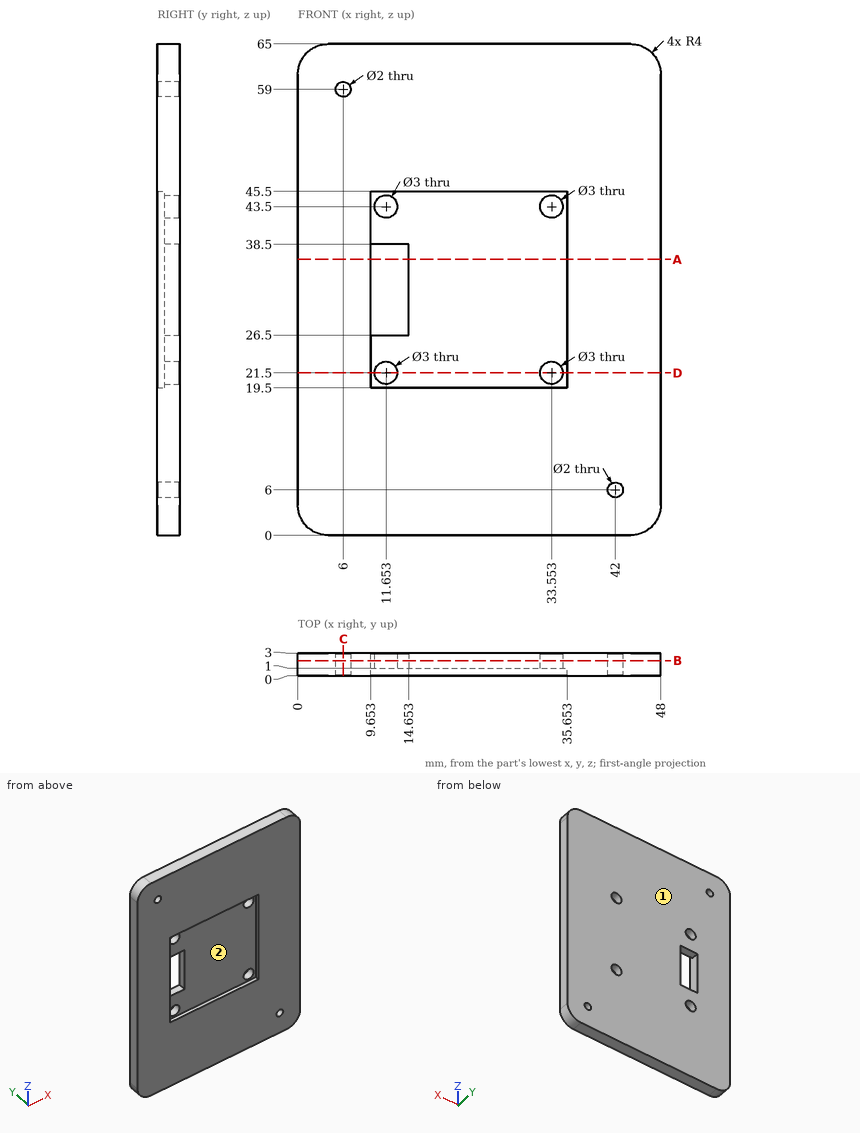
The figure shows three views and two pictorial views of one solid part (mm, origin at its lowest corner). Answer the questions. Give positions to 0.01 mm unless a question says otherwise; leave off trailing zeros. Loops run counter-clockwise (first coordinate to the right, second up) from the corner with the lowest first, then second, coordinate; pieces in that order, holes last. Notation, with made-up numbers: (71, 41) -> (81, 41) arc R23 ccw to (81, 50) -> close; hole circle Ø7 at (-15, 87). An arc over 180 degrees is marked (long way). Use a Markdown table: item, result. Add a question column.
1. Section C-C on x = 6 is taken. Determine the outline of the cut face in (y, z).
2. Section A-A on z = 36.5 is taken. Determine the outline of the cut face in (x, y).
3. Section B-B on y = 2.05 is taken. Determine the outline of the cut face in (x, z).
4. Section D-D on z = 21.5 is taken. Determine the outline of the cut face in (x, y).
5. Find the intervals of material crossed by probe 1 along X at (y, z) = (1.85, 43.5); probe 2 along Z at (x, y) = (42, 1.95); probe 3 along X at (y, z) = (0.95, 22.5), in increasing order.
6. Determine the mould class of the marked faces 1 and 2 for opening direction Z: released by +Z, released by -Z, zero draft, split by the parting line, or undercut.
Results below:
| question | item | result |
|---|---|---|
| 1 | outline | (0, 0) -> (3, 0) -> (3, 58) -> (0, 58) -> close; (0, 60) -> (3, 60) -> (3, 65) -> (0, 65) -> close |
| 2 | outline | (0, 0) -> (9.65, 0) -> (9.65, 3) -> (0, 3) -> close; (14.65, 1) -> (35.65, 1) -> (35.65, 0) -> (48, 0) -> (48, 3) -> (14.65, 3) -> close |
| 3 | outline | (0, 4) arc R4 ccw to (4, 0) -> (44, 0) arc R4 ccw to (48, 4) -> (48, 61) arc R4 ccw to (44, 65) -> (4, 65) arc R4 ccw to (0, 61) -> close; hole circle Ø2 at (6, 59); hole (9.65, 26.5) -> (14.65, 26.5) -> (14.65, 38.5) -> (9.65, 38.5) -> close; hole circle Ø3 at (11.65, 21.5); hole circle Ø3 at (11.65, 43.5); hole circle Ø3 at (33.55, 21.5); hole circle Ø3 at (33.55, 43.5); hole circle Ø2 at (42, 6) |
| 4 | outline | (0, 0) -> (9.65, 0) -> (9.65, 1) -> (10.15, 1) -> (10.15, 3) -> (0, 3) -> close; (13.15, 1) -> (32.05, 1) -> (32.05, 3) -> (13.15, 3) -> close; (35.05, 1) -> (35.65, 1) -> (35.65, 0) -> (48, 0) -> (48, 3) -> (35.05, 3) -> close |
| 5 | probe 1 | x = 0 to 10.15, 13.15 to 32.05, 35.05 to 48 |
| 5 | probe 2 | z = 0 to 5, 7 to 65 |
| 5 | probe 3 | x = 0 to 9.65, 35.65 to 48 |
| 6 | face 1 | zero draft |
| 6 | face 2 | undercut |
